```python
from build123d import *

# Parameters (mm, degrees)
F0_W     = 152.4
F0_H     = 127
F1_DEPTH = 127
F2_W     = 88.9
F2_H     = 88.9
F3_DEPTH = 88.9
F4_R     = 19.05
F5_DEPTH = 50.8
F6_W     = 38.1
F6_H     = 38.1
F7_DEPTH = 63.5
F8_SIZE  = 30.48
F9_R     = 38.1


with BuildPart() as f1:
    # F0 (on Front) → F1 (new body)
    with BuildSketch(Plane.XZ):
        Rectangle(F0_W, F0_H)
    extrude(amount=F1_DEPTH)

    # F2 (on face) → F3 (cut)
    with BuildSketch(Plane.XY.offset(63.5)):
        with Locations((31.75, -82.55)):
            Rectangle(F2_W, F2_H)
    extrude(amount=-F3_DEPTH, mode=Mode.SUBTRACT)

    # F4 (on face) → F5 (cut)
    with BuildSketch(Plane.XY.offset(-25.4)):
        with Locations((31.75, -82.55)):
            Circle(F4_R)
    extrude(amount=-F5_DEPTH, mode=Mode.SUBTRACT)

    # F6 (on face) → F7 (cut)
    with BuildSketch(Plane.XY.offset(63.5)):
        with Locations((6.35, -19.05)):
            Rectangle(F6_W, F6_H)
    extrude(amount=-F7_DEPTH, mode=Mode.SUBTRACT)

    # F8
    f8_edges = [f1.edges().sort_by_distance(p)[0] for p in [
        (76.2, -19.05, 63.5),
    ]]
    chamfer(f8_edges, length=F8_SIZE)

    # F9
    f9_edges = [f1.edges().sort_by_distance(p)[0] for p in [
        (-44.45, -127, 63.5),
    ]]
    fillet(f9_edges, radius=F9_R)


solid = f1.part
```
Verification items for the finished model (mm, model axes). A direction names the side the tool comes from. Coordinates: 2 decimals unless noted, no trailing zeros. Write each loop counter-clockwise with the first axis right and the second up, starting at its lowest first coordinate (ties: lowest second). Pieces come first, ordered by that corner, then holes. Notation, with made-up numbers: (75.5, 10) - (95.5, 10) arc R28 ccw to (95.5, 46) - close; hole circle Ø5 at (73.5, 59). An arc over 180 degrees is marked (long way). One line per question, with ' | ' between items. Start each with the question number.
1. Section check D-D (z = -31). Enter the section's corners in (x, y).
2. Section check B-B (y = -82.55). Enter the section's corners in (x, z).
3. Draft check along X on faces 4 (the flat face through (-76.2, -63, -1)), 5 (the flat face through (25.4, -19, 32)), 6 (the flat face through (35, -19, 63.5)), 7 (the flat face through (6, -19, 0)). Enter one of: released by +X, released by -X, zero draft, split by the parting line, or undercut.
4. Section check A-A (x = 31.75). Enter the section's corners in (y, z), plus the area to 3 significant figures.
5. Access from +Z, -Z, +X, -X, +Y, -Y to the whole of each face (thin tool, end or side, straight path). Record for faces 1 (the flat face through (-12.7, -64, 20)), 2 (the cylindrical face through (-44.01, -116.14, 52.04)), 3 (the flat face through (41, -38.1, 10)).
6. Section check C-C (z = 21). Enter the section's corners in (x, y).
7. Gauge pin test, flat ends, axial feed: P1, Ø11.5, axis at x = 0, y = -23, coming from the +Z side; P2, Ø12, axis at x = -57.5, z = -40, coming from the +Y side; P3, Ø1.5, axis at x = -37, y = -99, coming from the +Z side; P4, Ø4, axis at y = -45.5, z = -20, coming from the +X side. Record the tip position at first contact, or that the pin passes through.
8. Material ranges on line 1 along Y through (x, z) = (31.75, -52.5); line 2 along X through (y, z) = (-82, -48); line 3 along Z through (x, y) = (66, -50), recorded low to high.
Computed values:
1) outline: (-76.2, -127) - (76.2, -127) - (76.2, 0) - (-76.2, 0) - close; hole circle Ø38.1 at (31.75, -82.55)
2) outline: (-76.2, -63.5) - (12.7, -63.5) - (12.7, -25.4) - (-12.7, -25.4) - (-12.7, 63.5) - (-76.2, 63.5) - close; (50.8, -63.5) - (76.2, -63.5) - (76.2, -25.4) - (50.8, -25.4) - close
3) face 4: released by -X | face 5: undercut | face 6: zero draft | face 7: undercut
4) outline: (-127, -63.5) - (-101.6, -63.5) - (-101.6, -25.4) - (-127, -25.4) - close; (-63.5, -63.5) - (0, -63.5) - (0, 63.5) - (-38.1, 63.5) - (-38.1, -25.4) - (-63.5, -25.4) - close | area: 6,770 mm²
5) face 1: +Z, -Y | face 2: +Z, +X, -X, -Y | face 3: +Z, +X, -Y
6) outline: (-76.2, -127) - (-12.7, -127) - (-12.7, 0) - (-76.2, 0) - close; (25.4, -38.1) - (76.2, -38.1) - (76.2, 0) - (25.4, 0) - close
7) P1: z = 0 | P2: y = 0 | P3: z = 62.33 | P4: x = -12.7
8) line 1: -127 to -101.6, -63.5 to 0 | line 2: -76.2 to 12.71, 50.79 to 76.2 | line 3: -63.5 to -25.4
